The figure shows three views and two pictorial views of one solid part (mm, origin at its lowest corner). Answer the questions. Give positions to 0.01 mm unless a question says otherwise; leave off trailing zeros. Loops run counter-clockwise (first coordinate to the right, second up) from the corner with the lowest first, then second, coordinate; pieces in that order, holes last. Notation, with made-up numbers: (-35, 31.25) - (-9, 31.25) arc R31 cw to (-9, 64.25) - close; hole circle Ø3 at (-5, 67). An arc over 180 degrees is marked (long way). Use CSV: the item, a comma, the result in double quotes.
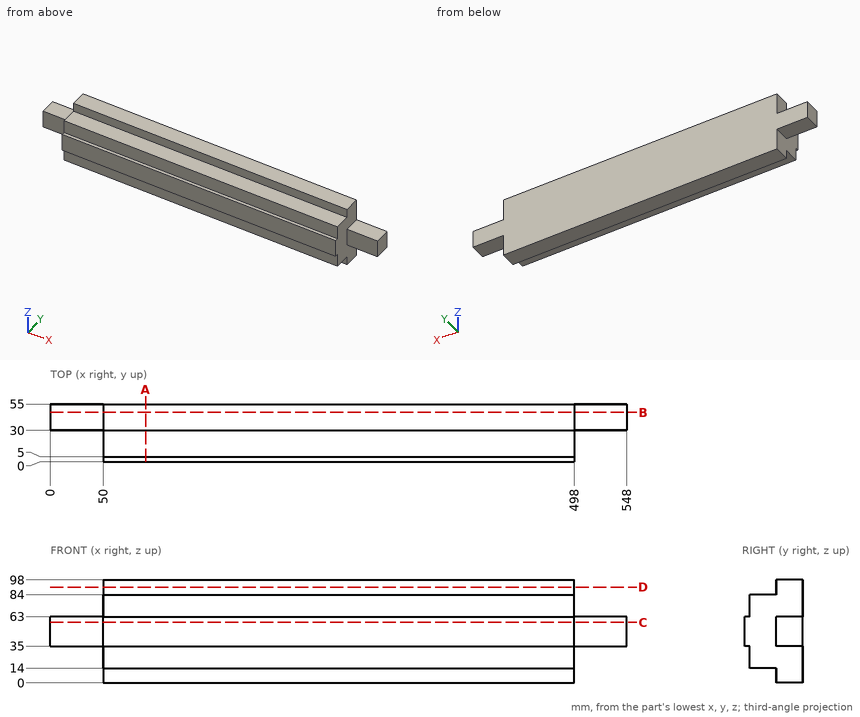
Item 1: A cutting plane is placed at A-A on x = 90.5. Determine the outline of the cut face in (y, z).
Determined:
outline,"(0, 35) - (5, 35) - (5, 14) - (30, 14) - (30, 0) - (55, 0) - (55, 98) - (30, 98) - (30, 84) - (5, 84) - (5, 63) - (0, 63) - close"
Item 2: Given P1, Ø7.5, axis at x = 299.5, y = 15, coming from the -Z side; P2, Ø12.5, axis at x = 28.5, y = 41, coming from the -Z side; P3, Ø4, axis at x = 321.5, y = 3.5, coming from the +Z side, each flat-ended and moving along its own axis, determine where each tip first touches the part or whether it passes through.
Determined:
P1,"stops at z = 14"
P2,"stops at z = 35"
P3,"stops at z = 84"
Item 3: A cutting plane is placed at C-C on z = 57.5. Determine the outline of the cut face in (x, y), and give its area (3 significant figures).
Determined:
outline,"(0, 30) - (50, 30) - (50, 0) - (498, 0) - (498, 30) - (548, 30) - (548, 55) - (0, 55) - close"
area,"27,100 mm²"
Item 4: A cutting plane is placed at B-B on y = 47. Determine the outline of the cut face in (x, z), and give its area (3 significant figures).
Determined:
outline,"(0, 35) - (50, 35) - (50, 0) - (498, 0) - (498, 35) - (548, 35) - (548, 63) - (498, 63) - (498, 98) - (50, 98) - (50, 63) - (0, 63) - close"
area,"46,700 mm²"
Item 5: Find the intervals of material crossed by line 1 (X direction, y = 35, z = 86); line 2 (Z direction, x = 315.5, y = 11); line 3 (Y direction, x = 463.5, z = 33), in increasing order.
Determined:
line 1,"x = 50 to 498"
line 2,"z = 14 to 84"
line 3,"y = 5 to 55"
Item 6: A cutting plane is placed at D-D on z = 91. Determine the outline of the cut face in (x, y), and give its area (3 significant figures).
Determined:
outline,"(50, 30) - (498, 30) - (498, 55) - (50, 55) - close"
area,"11,200 mm²"
